The drawing under review shows one solid part. Ordinate dimensions are in mm from its lowest x, y, z. Round coordinates to 2 decimals unless told otherwise and drop trailing zeros. Write each loop counter-clockwise with the first axis right and the second up, starting at its lowest first coordinate (ties: lowest second). Pieces come first, ordered by that corner, then holes. Notation, with made-up numbers: (44, -26) -> (87, -26) arc R7 ccw to (87, -13) -> close; hole circle Ø10 at (23, 64). An arc over 180 degrees is marked (long way). Answer in a Markdown table with one row per item.
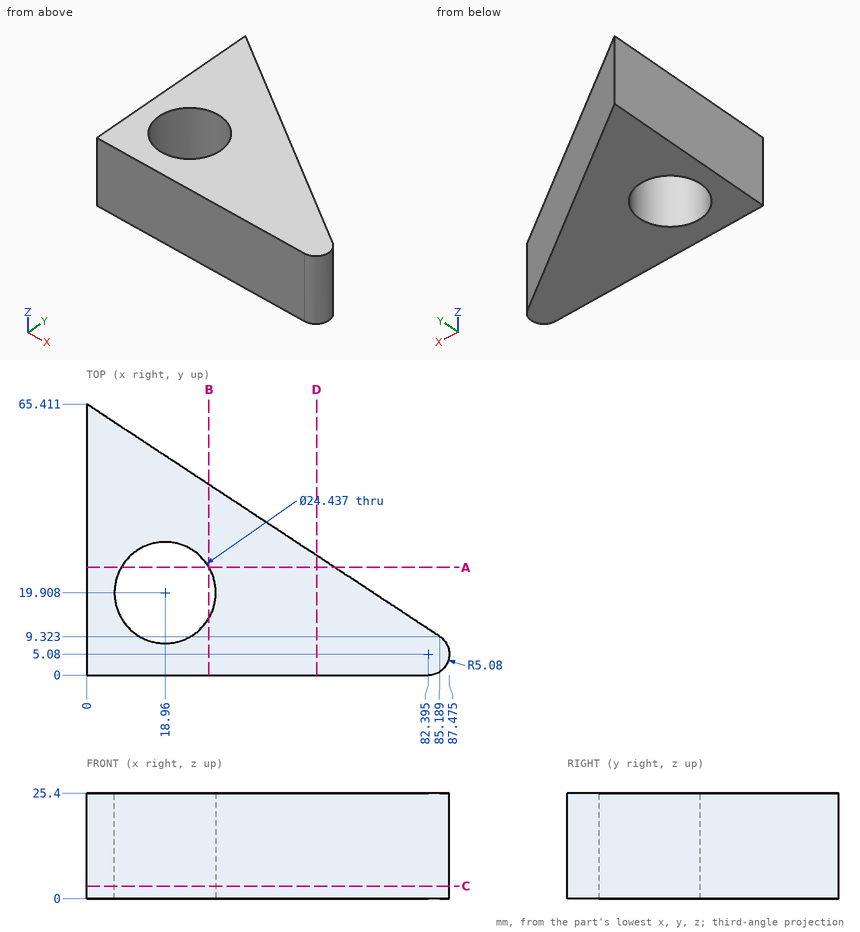
1) Consider section C-C on z = 3. State the section outline as (x, y) points (1 decimal), then the cut area to 3 significant figures.
Solved:
| item | result |
|---|---|
| outline | (0, 0) -> (82.4, 0) arc R5.1 ccw to (85.2, 9.3) -> (0, 65.4) -> close; hole circle Ø24.4 at (19, 19.9) |
| area | 2,730 mm² |
2) For line 1 (Y direction, x = 8.5, z = 8.75) (1 decimal); line 2 (Y direction, x = 9.5, z = 2.25) (1 decimal); line 3 (X direction, y = 25, z = 10.25) (1 decimal), list the stretches that pass through material, from the lowest coordinate up. Write a range as [from, to].
Solved:
| item | result |
|---|---|
| line 1 | [0, 13.6], [26.2, 59.8] |
| line 2 | [0, 12.2], [27.6, 59.2] |
| line 3 | [0, 7.9], [30.1, 61.4] |
3) Clearance check with flat-ended pins moving along their axes: pin 1 Ø6 at (x, z) = (19, 9.5) entering from +Y; pin 2 Ø2 at (y, z) = (36, 20.5) entering from +X. State where each tip first meets the part, or that it passes through.
Solved:
| item | result |
|---|---|
| pin 1 | y = 54.88 |
| pin 2 | x = 46.19 |
4) Consider section B-B on x = 29.5. State the section outline as (y, z) points.
Solved:
| item | result |
|---|---|
| outline | (0, 0) -> (13.73, 0) -> (13.73, 25.4) -> (0, 25.4) -> close; (26.09, 0) -> (45.99, 0) -> (45.99, 25.4) -> (26.09, 25.4) -> close |
5) Consider section D-D on x = 55.5. State the section outline as (y, z) points.
Solved:
| item | result |
|---|---|
| outline | (0, 0) -> (28.87, 0) -> (28.87, 25.4) -> (0, 25.4) -> close |
6) Consider section A-A on y = 26. State the section outline as (x, z) points.
Solved:
| item | result |
|---|---|
| outline | (0, 0) -> (8.37, 0) -> (8.37, 25.4) -> (0, 25.4) -> close; (29.55, 0) -> (59.86, 0) -> (59.86, 25.4) -> (29.55, 25.4) -> close |
